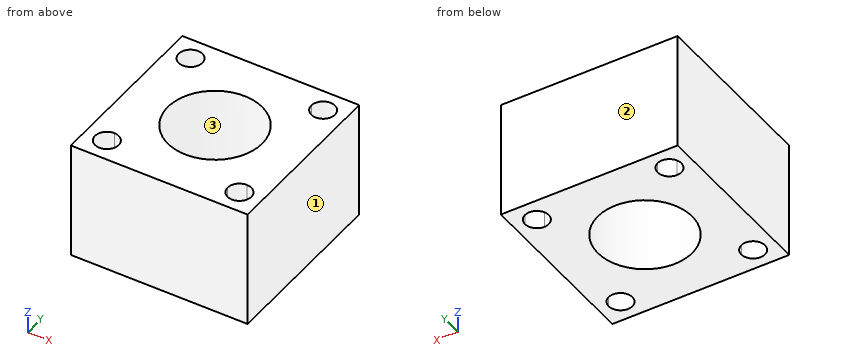
```python
from build123d import *

# Parameters (mm, degrees)
F0_W     = 25.4
F0_H     = 14.2875
F1_DEPTH = 25.4
F2_R     = 10.16
F3_DEPTH = 25.401
F5_DEPTH = 25.401


# Not quite as in the source:
# - a feature names something its author has since deleted; it is built from what else it names


with BuildPart() as f1:
    # F0 (on Top) → F1 (new body)
    with BuildSketch(Plane.XY):
        with Locations((-34.7179355979, 53.2439169049)):
            Rectangle(F0_W, F0_H)
        Polygon((-22.0179355979, 46.1001669049), (-47.4179355979, 46.1001669049), (-47.4179355979, -30.0998330951), (-22.0179355979, -30.0998330951), (54.1820644021, -30.0998330951), (54.1820644021, 46.1001669049), align=None)
        with Locations((-34.7179355979, -37.2435830951)):
            Rectangle(F0_W, F0_H)
    extrude(amount=F1_DEPTH)

    # F2 (on face) → F3 (cut, through all)
    with BuildSketch(Plane.XY.offset(25.4)):
        with Locations((35.1320644021, 8.0001669049)):
            Circle(F2_R)
        with BuildLine():
            Line((23.3972644021, 22.2876669049), (20.8445644021, 22.2876669049))
            Line((20.8445644021, 22.2876669049), (20.8445644021, 19.7349669049))
            ThreePointArc((20.8445644021, 19.7349669049), (22.6495958824, 20.4826354246), (23.3972644021, 22.2876669049))
        make_face()
        with BuildLine():
            Line((20.8445644021, 19.7349669049), (20.8445644021, 22.2876669049))
            Line((20.8445644021, 22.2876669049), (23.3972644021, 22.2876669049))
            ThreePointArc((23.3972644021, 22.2876669049), (19.0395329218, 24.0926983853), (20.8445644021, 19.7349669049))
        make_face()
        with BuildLine():
            ThreePointArc((51.9722644021, 22.2876669049), (49.4195644021, 24.8403669049), (46.8668644021, 22.2876669049))
            Line((46.8668644021, 22.2876669049), (49.4195644021, 22.2876669049))
            Line((49.4195644021, 22.2876669049), (49.4195644021, 19.7349669049))
            ThreePointArc((49.4195644021, 19.7349669049), (51.2245958824, 20.4826354246), (51.9722644021, 22.2876669049))
        make_face()
        with BuildLine():
            Line((49.4195644021, 22.2876669049), (46.8668644021, 22.2876669049))
            ThreePointArc((46.8668644021, 22.2876669049), (47.6145329218, 20.4826354246), (49.4195644021, 19.7349669049))
            Line((49.4195644021, 19.7349669049), (49.4195644021, 22.2876669049))
        make_face()
        with BuildLine():
            Line((49.4195644021, -6.2873330951), (49.4195644021, -3.7346330951))
            ThreePointArc((49.4195644021, -3.7346330951), (47.6145329218, -4.4823016147), (46.8668644021, -6.2873330951))
            Line((46.8668644021, -6.2873330951), (49.4195644021, -6.2873330951))
        make_face()
        with BuildLine():
            ThreePointArc((51.9722644021, -6.2873330951), (51.2245958824, -4.4823016147), (49.4195644021, -3.7346330951))
            Line((49.4195644021, -3.7346330951), (49.4195644021, -6.2873330951))
            Line((49.4195644021, -6.2873330951), (46.8668644021, -6.2873330951))
            ThreePointArc((46.8668644021, -6.2873330951), (49.4195644021, -8.8400330951), (51.9722644021, -6.2873330951))
        make_face()
        with BuildLine():
            ThreePointArc((23.3972644021, -6.2873330951), (22.6495958824, -4.4823016147), (20.8445644021, -3.7346330951))
            Line((20.8445644021, -3.7346330951), (20.8445644021, -6.2873330951))
            Line((20.8445644021, -6.2873330951), (23.3972644021, -6.2873330951))
        make_face()
        with BuildLine():
            Line((20.8445644021, -6.2873330951), (20.8445644021, -3.7346330951))
            ThreePointArc((20.8445644021, -3.7346330951), (19.0395329218, -8.0923645754), (23.3972644021, -6.2873330951))
            Line((23.3972644021, -6.2873330951), (20.8445644021, -6.2873330951))
        make_face()
    extrude(amount=-F3_DEPTH, mode=Mode.SUBTRACT)

    # F4 (on face) → F5 (cut, through all)
    with BuildSketch(Plane.XY.offset(25.4)):
        Polygon((54.1820644021, -30.0998330951), (54.1820644021, -11.0498330951), (16.0820644021, -11.0498330951), (16.0820644021, 27.0501669049), (54.1820644021, 27.0501669049), (54.1820644021, 46.1001669049), (-22.0179355979, 46.1001669049), (-22.0179355979, 60.3876669049), (-47.4179355979, 60.3876669049), (-47.4179355979, -44.3873330951), (-22.0179355979, -44.3873330951), (-22.0179355979, -30.0998330951), align=None)
    extrude(amount=-F5_DEPTH, mode=Mode.SUBTRACT)


solid = f1.part
```
The model under review builds one solid part; all positions refer to its coordinate system, in mm. Face numbers are marked on the shaded views. Give positions to 0.01 mm unless a question says otherwise; leave off trailing zeros. Write each loop counter-clockwise with the first axis right and the second up, starting at its lowest first coordinate (ties: lowest second). Pieces come first, ordered by that corner, then holes. Notation, with made-up numbers: M -15.75,27.25 L 39.25,27.25 A28 ccw 39.25,58.25 Z; hole C 61,8 d5. An arc over 180 degrees is marked long. Write item = value, one per line. Start each with the question number.
Q1. We need section A-A (x = 50.5). State the section outline as (y, z) points, plus the area to 3 significant figures.
Q2. For line 1 (Y direction, x = 21, z = 6.5); line 2 (Y direction, x = 50, z = 17); line 3 (X direction, y = 23.5, z = 6.75), list the stretches that pass through material, from the lowest coordinate up.
Q3. Mouldability with a two-part tool opening along X and no side actions: class the marked faces 1, 2 and 3 as released by +X, released by -X, zero draft, split by the parting line, or undercut.
Q4. We need section C-C (z = 21.25). State the section outline as (x, y) points.
Q5. We need section D-D (x = 29.5). State the section outline as (y, z) points, plus the area to 3 significant figures.
Q6. We need section B-B (y = 0.5). State the section outline as (x, z) points, plus the area to 3 significant figures.
Result set:
q1.outline = M -11.05,0 L -8.6,0 L -8.6,25.4 L -11.05,25.4 Z; M -3.97,0 L 19.97,0 L 19.97,25.4 L -3.97,25.4 Z; M 24.6,0 L 27.05,0 L 27.05,25.4 L 24.6,25.4 Z
q1.area = 733 mm2
q2.line_1 = -11.05 to -8.84, -3.74 to 19.74, 24.84 to 27.05
q2.line_2 = -11.05 to -8.77, -3.8 to 19.8, 24.77 to 27.05
q2.line_3 = 16.08 to 18.6, 23.09 to 47.17, 51.67 to 54.18
q3.face_1 = released by +X
q3.face_2 = zero draft
q3.face_3 = undercut
q4.outline = M 16.08,-11.05 L 54.18,-11.05 L 54.18,27.05 L 16.08,27.05 Z; hole C 20.84,-6.29 d5.11; hole C 20.84,22.29 d5.11; hole C 35.13,8 d20.32; hole C 49.42,-6.29 d5.11; hole C 49.42,22.29 d5.11
q5.outline = M -11.05,0 L -0.46,0 L -0.46,25.4 L -11.05,25.4 Z; M 16.46,0 L 27.05,0 L 27.05,25.4 L 16.46,25.4 Z
q5.area = 538 mm2
q6.outline = M 16.08,0 L 28.28,0 L 28.28,25.4 L 16.08,25.4 Z; M 41.99,0 L 54.18,0 L 54.18,25.4 L 41.99,25.4 Z
q6.area = 620 mm2
